```python
from build123d import *

# Parameters (mm, degrees)
BOSS_EXTRUDE1_DEPTH = 10


with BuildPart() as part:
    # Sketch2 → Boss-Extrude1 (new body)
    with BuildSketch(Plane(origin=(0, 0, 0), x_dir=(1, 0, 0), z_dir=(0, 1, 0))):
        with BuildLine():
            Line((4.267766953, 76.762899821), (76.762899821, 4.267766953))
            ThreePointArc((76.762899821, 4.267766953), (77.304831699, 1.543291419), (74.995132868, 0))
            Line((74.995132868, 0), (2.5, 0))
            ThreePointArc((2.5, 0), (0.732233047, 0.732233047), (0, 2.5))
            Line((0, 2.5), (0, 74.995132868))
            ThreePointArc((0, 74.995132868), (1.543291419, 77.304831699), (4.267766953, 76.762899821))
        make_face()
    extrude(amount=BOSS_EXTRUDE1_DEPTH)


solid = part.part
```
Model file for the job. Use its own axes, mm. Give positions to 0.01 mm unless a question says otherwise; leave off trailing zeros. Write each loop counter-clockwise with the first axis right and the second up, starting at its lowest first coordinate (ties: lowest second). Pieces come first, ordered by that corner, then holes. Notation, with made-up numbers: (83.25, 18) - (130.25, 18) arc R16 ccw to (130.25, 44) - close; hole circle Ø7 at (78.25, 77). An arc over 180 degrees is marked (long way). One line per question, with ' | ' between items. Start each with the question number.
(1) Slice it at C-C on x = 13.5. Write the cut outline in (y, z), plus the area to 3 significant figures.
(2) Pin check, flat tips, straight feed: P1, Ø1.5, axis at y = 3.5, z = -63.5, coming from the +X side; P2, Ø6, axis at y = 7.5, z = -36, coming from the +X side. Stop position of each tip, or through.
(3) Wall check: line 1 along Z through (x, y) = (66.5, 2.5); line 2 along X through (y, z) = (8.25, -35); line 3 along X through (y, z) = (8, -64.5). Give the ranges that are in metal, low to high. Write a range as from..to.
(4) Slice it at A-A on y = 4.25. Write the cut outline in (x, z).
(5) Two-plate mould, pull along X, no slides. Class faces 1 (the face through (39, 5, 0)), 2 (the face through (40.01, 4.93, -41.02)), 3 (the face through (0.752, 4.93, -0.713)): +X half, -X half, draft (parallel to the pull), parting line (faces both ways), or undercut.
(6) Slice it at B-B on z = -50.5. Write the cut outline in (x, y).
Results below:
1) outline: (0, -67.53) - (10, -67.53) - (10, 0) - (0, 0) - close | area: 675 mm^2
2) P1: x = 18.28 | P2: x = 48.03
3) line 1: -14.53..0 | line 2: 0..46.03 | line 3: 0..16.53
4) outline: (0, -75) arc R2.5 ccw to (4.27, -76.76) - (76.76, -4.27) arc R2.5 ccw to (75, 0) - (2.5, 0) arc R2.5 ccw to (0, -2.5) - close
5) face 1: draft | face 2: +X half | face 3: -X half
6) outline: (0, 0) - (30.53, 0) - (30.53, 10) - (0, 10) - close
